Source: CAD feature listing. Evaluate the final solid. Frame: model axes, mm. A direction names the side the tool comes from. Give positions to 0.01 mm unless a question says otherwise; leave off trailing zeros. Order: outer loops, then holes, each group sorted by start corner. A loop starts at its lowest first (then second) coordinate and runs counter-clockwise, first axis right, second up. Notation, with made-up numbers: M 62.5,-4 L 84.5,-4 A20 ccw 84.5,30 Z; hole C 11.5,61 d3. An arc over 180 degrees is marked long. Answer in a Markdown table with one row per item. Add a question column.
(1) Set-up query: faces 4 (the face through (14.65, -0.54, 2.44)), 5 (the face through (-2.75, -2, 0)), 6 (the face through (-2, 1.5, 0)). Return all of +Z, -Z, +X, -X, +Y, -Y with unobstructed straight access to the full face (end or side cutting, diameter ignored); none if empty.
(2) Material intervals for line 1 along Z through (x, y) = (23, 0); line 2 along X through (y, z) = (0.25, 2); line 3 along Y through (x, z) = (7.5, 1.5), sorted ascending.
(3) Mould query, pull axis Y, two halves, no side actions, for faces 1 (the face through (-0.193, 2.192, 4.214)), 2 (the face through (30, 0, 0)), 3 (the face through (-2, -1.5, 0)). Classes: pulls with the +Y half, pulls with the -Y half, needs draft (parallel to the pull), parting line crosses it, or undercut.
(4) Pin query (flat end, axial travel): P1, Ø2, axis at x = 14, y = -0.5, coming from the -Z side; P2, Ø0.8, axis at x = -1.5, z = 0.5, coming from the +Y side; P3, Ø1, axis at x = 3, z = -0.5, coming from the -Y side. Return the tip coordinate at first contact, or that it passes through.
(5) Section query A-A, the plane x = 0.5. Return loops of the section in (y, z).
Autodesk Inventor part; units mm, degrees
ref_plane "Work Plane1" through (29, 0, 0) normal (0, -1, 0) x (1, 0, 0)
ref_plane "YZ Plane" through (0, 0, 0) normal (1, 0, 0) x (0, 1, 0)
ref_plane "XZ Plane" through (0, 0, 0) normal (0, 1, 0) x (-1, 0, 0)
sketch "Sketch1" plane through (0, 0, 0) normal (0, 0, 1) x (1, 0, 0)
  line L0 (-0.19, 0) -> (30, 0)
  line L1 (30, 0) -> (30, 2.5)
  line L2 (30, 2.5) -> (8, 2.5)
  line L3 (8, 2.5) -> (7.5091, 2.5)
  line L4 (7.5091, 2.5) -> (0, 2.5)
  line L5 (0, 2.5) -> (0, 4.75)
  line L6 (0, 4.75) -> (-2.75, 4.75)
  line L7 (-2.75, 4.75) -> (-2.75, 1.7321)
  line L8 (-2.75, 1.7321) -> (-1.19, 1.7321)
  line L9 (-1.19, 1.7321) -> (-0.19, 0)
  line L10 (-9.3, 0) -> (36.55, 0)
  line L11 (0, -0.95) -> (0, 5.7)
  line L12 (8, 2.5) -> (0, 2.5) construction
  dimension "d1" = 22
  dimension "d2" = 0.4909
  dimension "d3" = 2.75
  dimension "d4" = 1.56
  dimension "d5" = 60
  dimension "d6" = 5
  dimension "d7" = 5
  dimension "d8" = 3.4641
  dimension "d9" = 9.5
  dimension "d26" = 30
revolve "Body" add sketch "Sketch1" angle 360 about axis through (-0.19, 0, 0) along (1, 0, 0)
sketch "Sketch2" plane through (-2.75, 0, 0) normal (-1, 0, 0) x (0, 0, 1)
  circle A0 centre (0, 0) radius 1.7321
  line L0 (0, -6.65) -> (0, 6.65)
  line L1 (-6.65, 0) -> (6.65, 0)
  line L2 (1.7321, 0) -> (0.866, -1.5)
  line L3 (0.866, -1.5) -> (-0.866, -1.5)
  line L4 (-0.866, -1.5) -> (-1.7321, 0)
  line L5 (-1.7321, 0) -> (-0.866, 1.5)
  line L6 (-0.866, 1.5) -> (0.866, 1.5)
  line L7 (0.866, 1.5) -> (1.7321, 0)
extrude "Slot" add sketch "Sketch2" against normal up to next contours L7 A0 | A0 L2 | L6 L0 A0 | A0 L0 L3 | L0 L6 A0 | A0 L3 L0 | L4 A0 | A0 L5
fillet "Fillet1" radius 2.37 1 edges at (-2.75, -4.75, 0)
thread "Thread"
chamfer "Chamfer1" distance 0.4908 distance2 0.4908 1 edges at (30, -2.5, 0) measured on face at (30, -0.5525, -0.0341)
ref_plane "Work Plane1" through (29, 0, 0) normal (0, -1, 0) x (1, 0, 0)
fillet "Fillet2" radius 0.2 1 edges at (0, -2.5, 0)
equation "\"d1\" = GEL"
equation "\"d3\" = KOH"
equation "\"d4\" = INTI"
equation "\"d6\" = GD"
equation "\"d7\" = BDM"
equation "\"d8\" = 1.1547 * SW"
equation "\"d9\" = KOD"
equation "\"d26\" = NLG"
equation "\"d30\" = R"
equation "\"d17\" = RR"
equation "\"d13\" = GEL"
equation "\"d15\" = -0.5 * SPD + 0.5 * GD"
equation "\"d16\" = GUL"
equation "\"GD\" = NND"
equation "\"NLG\" = 30"
equation "\"GEL\" = 22"
equation "\"KOD\" = 9.5"
equation "\"KOH\" = 2.75"
equation "\"INTI\" = 1.56"
equation "\"GAL\" = 0.61345 * PTC"
equation "\"GUL\" = 0.61345 * PTC"
equation "\"BDM\" = NND"
equation "\"SW\" = 3"
equation "\"RR\" = 2.37"
equation "\"SPD\" = NND - 1.2269 * PTC"
equation "\"R\" = 0.2"
equation "\"TOA\" = 30deg"
equation "\"GD1\" = THREADDIA - 1.2269 * PTC"
equation "\"THREADDIA\" = 5"
equation "\"PTC\" = 0.8"
equation "\"NND\" = 5"
equation "\"KOH1\" = 0.38"
equation "\"E0\" = 3.443"
properties part number "ISO 7380-1 - M5 x 30" material "Steel"
Values follow:
| question | item | result |
|---|---|---|
| 1 | face 4 | +X |
| 1 | face 5 | +Z, -Z, -X, +Y, -Y |
| 1 | face 6 | -X |
| 2 | line 1 | z = -2.5 to 2.5 |
| 2 | line 2 | x = -2.75 to 29.99 |
| 2 | line 3 | y = -2 to 2 |
| 3 | face 1 | parting line crosses it |
| 3 | face 2 | needs draft |
| 3 | face 3 | undercut |
| 4 | P1 | stops at z = -2.5 |
| 4 | P2 | stops at y = 4.62 |
| 4 | P3 | stops at y = -2.5 |
| 5 | outline | C 0,0 d5 |
